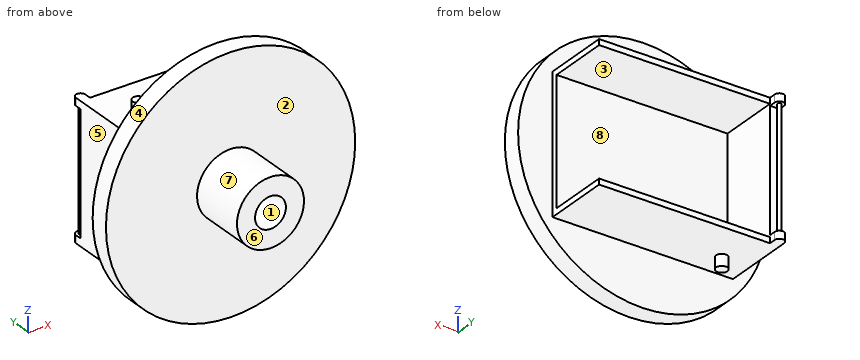
```python
from build123d import *

# Parameters (mm, degrees)
SKETCH1_W           = 95
SKETCH1_H           = 72
BOSS_EXTRUDE1_DEPTH = 35
SKETCH5_W           = 90
SKETCH5_H           = 66
CUT_EXTRUDE1_DEPTH  = 32
SKETCH9_R           = 3
BOSS_EXTRUDE4_DEPTH = 6
BOSS_EXTRUDE5_DEPTH = 4
SKETCH11_R          = 65.611758171
BOSS_EXTRUDE6_DEPTH = 10
SKETCH12_R          = 17.640424805
SKETCH12_R_2        = 8.122416637
BOSS_EXTRUDE7_DEPTH = 30
SKETCH13_R          = 1
BOSS_EXTRUDE8_DEPTH = 68


with BuildPart() as part:
    # Sketch1 → Boss-Extrude1 (new body)
    with BuildSketch(Plane(origin=(0, 0, 0), x_dir=(1, 0, 0), z_dir=(0, 1, 0))):
        Rectangle(SKETCH1_W, SKETCH1_H)
    extrude(amount=BOSS_EXTRUDE1_DEPTH)

    # Sketch5 → Cut-Extrude1 (cut)
    with BuildSketch(Plane(origin=(0, 35, 0), x_dir=(1, 0, 0), z_dir=(0, 1, 0))):
        with Locations((2.5, 0)):
            Rectangle(SKETCH5_W, SKETCH5_H)
    extrude(amount=-CUT_EXTRUDE1_DEPTH, mode=Mode.SUBTRACT)

    # Sketch9 → Boss-Extrude4 (add)
    with BuildSketch(Plane.XY.offset(36)):
        with Locations(Location((-32.5, 13, 0), (0, 0, 180))):
            Circle(SKETCH9_R)
    boss_extrude4 = extrude(amount=BOSS_EXTRUDE4_DEPTH)

    # Mirror3: Boss-Extrude4 across plane
    add(boss_extrude4.mirror(Plane.XY))

    # Sketch10 → Boss-Extrude5 (add)
    with BuildSketch(Plane.XY.offset(36)):
        with BuildLine():
            Line((-42.5, 35), (-42.5, 38.5))
            ThreePointArc((-42.5, 38.5), (-45, 41), (-47.5, 38.5))
            Line((-47.5, 38.5), (-47.5, 35))
            Line((-47.5, 35), (-42.5, 35))
        make_face()
    boss_extrude5 = extrude(amount=-BOSS_EXTRUDE5_DEPTH)

    # Mirror4: Boss-Extrude5 across plane
    add(boss_extrude5.mirror(Plane.XY))

    # Sketch11 → Boss-Extrude6 (add)
    with BuildSketch(Plane.XZ):
        with Locations(Location((0, 0, 0), (0, 0, 270))):
            Circle(SKETCH11_R)
    extrude(amount=BOSS_EXTRUDE6_DEPTH)

    # Sketch12 → Boss-Extrude7 (add)
    with BuildSketch(Plane.XZ.offset(10)):
        with Locations(Location((0, 0, 0), (0, 0, 270))):
            Circle(SKETCH12_R)
        with Locations(Location((0, 0, 0), (0, 0, 270))):
            Circle(SKETCH12_R_2, mode=Mode.SUBTRACT)
    extrude(amount=BOSS_EXTRUDE7_DEPTH)

    # Sketch13 → Boss-Extrude8 (add)
    with BuildSketch(Plane.XY.offset(36)):
        with Locations((-45, 38.5)):
            Circle(SKETCH13_R)
    extrude(amount=-BOSS_EXTRUDE8_DEPTH)


solid = part.part
```
Check sheet for the modelled part. Datum: model origin and axes. Units: mm. Face numbers are marked on the shaded views. A direction names the side the tool comes from. Round coordinates to 2 decimals unless told otherwise and drop trailing zeros. Order: outer loops, then holes, each group sorted by start corner. A loop starts at its lowest first (then second) coordinate and runs counter-clockwise, first axis right, second up.
1) Scan lines: line 1 (X direction, y = -26, z = 0); line 2 (X direction, y = 18.5, z = -32.5); line 3 (Y direction, x = -8, z = -21). Record each from-to range of solid material in increasing order.
2) Section check A-A (z = 0). Record the boundary of the cut face in (x, y).
3) Section check B-B (x = 0). Record the boundary of the cut face in (y, z), and give its area (3 significant figures).
4) Section check C-C (y = 13). Record the boundary of the cut face in (x, z), and give its area (3 significant figures).
5) Mould release check, pull along Z, two halves, no side actions. Record for the marked faces 1, 2, 3 and 4: +Z half, -Z half, draft (parallel to the pull), parting line (faces both ways), or undercut.
6) Tool access check on the marked faces 5, 6, 7 and 8. Record the directions out of +Z, -Z, +X, -X, +Y, -Y that give a thin tool (end or side, any length) a straight path to the whole face; none if there is none.
7) Go/stop test with flat-tipped pins: pin 1 Ø4 at (x, y) = (-44, 39.5) entering from +Z; pin 2 Ø1.5 at (y, z) = (16.5, 11) entering from +X; pin 3 Ø4 at (x, z) = (21.5, -46) entering from +Y. Record where each tip stops, or that it passes through.
8) Section check D-D (z = 23.5). Record the boundary of the cut face in (x, y), and give its area (3 significant figures).
Result:
1. line 1: x = -17.64 to -8.12, 8.12 to 17.64
1. line 2: x = -47.5 to -42.5
1. line 3: y = -10 to 3
2. outline: (-65.61, -10) - (-17.64, -10) - (-17.64, -40) - (-8.12, -40) - (-8.12, -10) - (8.12, -10) - (8.12, -40) - (17.64, -40) - (17.64, -10) - (65.61, -10) - (65.61, 0) - (47.5, 0) - (47.5, 3) - (-42.5, 3) - (-42.5, 35) - (-47.5, 35) - (-47.5, 0) - (-65.61, 0) - close; circle Ø2 at (-45, 38.5)
3. outline: (-40, -17.64) - (-10, -17.64) - (-10, -65.61) - (0, -65.61) - (0, -36) - (35, -36) - (35, -33) - (3, -33) - (3, 33) - (35, 33) - (35, 36) - (0, 36) - (0, 65.61) - (-10, 65.61) - (-10, 17.64) - (-40, 17.64) - (-40, 8.12) - (-10, 8.12) - (-10, -8.12) - (-40, -8.12) - close
3. area: 2,290 mm2
4. outline: (-47.5, -36) - (-35.5, -36) - (-35.5, -42) - (-29.5, -42) - (-29.5, -36) - (47.5, -36) - (47.5, -33) - (-42.5, -33) - (-42.5, 33) - (47.5, 33) - (47.5, 36) - (-29.5, 36) - (-29.5, 42) - (-35.5, 42) - (-35.5, 36) - (-47.5, 36) - close
4. area: 972 mm2
5. face 1: undercut
5. face 2: draft
5. face 3: undercut
5. face 4: parting line
6. face 5: +Z, -Z, -X, +Y
6. face 6: +Z, -Z, +X, -X, -Y
6. face 7: -Y
6. face 8: +X, +Y
7. pin 1: stops at z = 36
7. pin 2: stops at x = -42.5
7. pin 3: stops at y = 0
8. outline: (-61.26, -10) - (61.26, -10) - (61.26, 0) - (47.5, 0) - (47.5, 3) - (-42.5, 3) - (-42.5, 35) - (-47.5, 35) - (-47.5, 0) - (-61.26, 0) - close; circle Ø2 at (-45, 38.5)
8. area: 1,670 mm2
